Input: part model. Units: mm. Frame: model coordinates. Coordinates: 2 decimals unless noted, no trailing zeros. Loops run counter-clockwise (first coordinate to the right, second up) from the corner with the lowest first, then second, coordinate; pieces in that order, holes last. Notation, with made-up numbers: (47.25, 57.25) -> (105.25, 57.25) arc R17 ccw to (105.25, 61.25) -> close; hole circle Ø7 at (-40, -37.5). An arc over 180 degrees is marked (long way). Answer as a JSON object with one key per item and string values.
from build123d import *

# Parameters (mm, degrees)
SKETCH2_W               = 60.452
SKETCH2_H               = 3.175
BOSS_EXTRUDE3_DEPTH     = 2.54
CUT_EXTRUDE2_DEPTH      = 361.893602522
CUT_EXTRUDE2_DEPTH_BACK = 361.893602522
SKETCH4_W               = 60.325
SKETCH4_H               = 3.175
SKETCH4_W_2             = 3.175
SKETCH4_H_2             = 31.75


with BuildPart() as part:
    # Sketch2 → Boss-Extrude3 (new body)
    with BuildSketch(Plane.XY):
        Polygon((-213.36, -244.2845), (-213.36, -263.2075), (-213.36, -269.6845), (-113.03, -269.6845), (-113.03, -244.2845), (132.334, -244.2845), (132.334, -241.1095), (192.786, -241.1095), (192.786, -244.2845), (213.36, -244.2845), (239.808280092, -244.2845), (239.808280092, -147.0025), (213.36, -147.0025), (213.36, 147.0025), (239.808280092, 147.0025), (239.808280092, 244.2845), (213.36, 244.2845), (192.786, 244.2845), (192.786, 241.1095), (132.334, 241.1095), (132.334, 244.2845), (-113.03, 244.2845), (-113.03, 269.6845), (-213.36, 269.6845), (-213.36, 244.2845), align=None)
        with Locations((-162.56, -242.697)):
            Rectangle(SKETCH2_W, SKETCH2_H, mode=Mode.SUBTRACT)
        with Locations((-162.56, 242.697)):
            Rectangle(SKETCH2_W, SKETCH2_H, mode=Mode.SUBTRACT)
    extrude(amount=BOSS_EXTRUDE3_DEPTH)

    # Sketch4 → Cut-Extrude2 (cut, two sides: drawn at the far end of the back side and taken through both)
    with BuildSketch(Plane.XY.offset(2.54).offset(-CUT_EXTRUDE2_DEPTH_BACK)):
        with Locations((-162.6235, -145.542)):
            Rectangle(SKETCH4_W, SKETCH4_H)
        with Locations((-162.6235, -48.471666667)):
            Rectangle(SKETCH4_W, SKETCH4_H)
        with Locations((-162.6235, 48.598666667)):
            Rectangle(SKETCH4_W, SKETCH4_H)
        with Locations((-162.6235, 145.669)):
            Rectangle(SKETCH4_W, SKETCH4_H)
        with Locations((162.6235, -145.542)):
            Rectangle(SKETCH4_W, SKETCH4_H)
        with Locations((162.6235, -48.471666667)):
            Rectangle(SKETCH4_W, SKETCH4_H)
        with Locations((162.6235, 48.598666667)):
            Rectangle(SKETCH4_W, SKETCH4_H)
        with Locations((162.6235, 145.669)):
            Rectangle(SKETCH4_W, SKETCH4_H)
        with Locations((211.7725, -194.056)):
            Rectangle(SKETCH4_W_2, SKETCH4_H_2)
        with Locations((211.7725, -97.028)):
            Rectangle(SKETCH4_W_2, SKETCH4_H_2)
        with Locations((211.7725, 0)):
            Rectangle(SKETCH4_W_2, SKETCH4_H_2)
        with Locations((211.7725, 97.028)):
            Rectangle(SKETCH4_W_2, SKETCH4_H_2)
        with Locations((211.7725, 194.056)):
            Rectangle(SKETCH4_W_2, SKETCH4_H_2)
        with Locations((-211.7725, -97.028)):
            Rectangle(SKETCH4_W_2, SKETCH4_H_2)
        with Locations((-211.7725, 0)):
            Rectangle(SKETCH4_W_2, SKETCH4_H_2)
        with Locations((-211.7725, -194.056)):
            Rectangle(SKETCH4_W_2, SKETCH4_H_2)
        with Locations((-211.7725, 97.028)):
            Rectangle(SKETCH4_W_2, SKETCH4_H_2)
        with Locations((-211.7725, 194.056)):
            Rectangle(SKETCH4_W_2, SKETCH4_H_2)
    extrude(amount=CUT_EXTRUDE2_DEPTH + CUT_EXTRUDE2_DEPTH_BACK, mode=Mode.SUBTRACT)


solid = part.part
1. Line query: line 1 along Y through (x, z) = (180.5, 0.8); line 2 along X through (y, z) = (48, 2); line 3 along Y through (x, z) = (103.5, 0.65). Output: solid intervals per line, ascending.
Reply:
{"line 1": "y = -241.11 to -147.13, -143.95 to -50.06, -46.88 to 47.01, 50.19 to 144.08, 147.26 to 241.11", "line 2": "x = -213.36 to -192.79, -132.46 to 132.46, 192.79 to 213.36", "line 3": "y = -244.28 to 244.28"}
2. Section query B-B (x = 185.5). Return loops of the section in (y, z), plus the area to 3 significant figures.
Reply:
{"outline": "(-241.11, 0) -> (-147.13, 0) -> (-147.13, 2.54) -> (-241.11, 2.54) -> close; (-143.95, 0) -> (-50.06, 0) -> (-50.06, 2.54) -> (-143.95, 2.54) -> close; (-46.88, 0) -> (47.01, 0) -> (47.01, 2.54) -> (-46.88, 2.54) -> close; (50.19, 0) -> (144.08, 0) -> (144.08, 2.54) -> (50.19, 2.54) -> close; (147.26, 0) -> (241.11, 0) -> (241.11, 2.54) -> (147.26, 2.54) -> close", "area": "1,190 mm2"}
3. Section query C-C (z = 0.7). Count the separate pieces of the cut face and the enclosed holes in it, plus the area to 3 significant figures.
Reply:
{"separate pieces": "1", "enclosed holes": "12", "area": "215,000 mm2"}
4. Section query D-D (y = -74). Return loops of the section in (x, z), plus the area to 3 significant figures.
Reply:
{"outline": "(-213.36, 0) -> (213.36, 0) -> (213.36, 2.54) -> (-213.36, 2.54) -> close", "area": "1,080 mm2"}
5. Pin query (flat end, axial travel): P1, Ø1.3, axis at x = 212.5, z = 1, coming from the +Y side; P2, Ø1.3, axis at x = 174, z = 2, coming from the -Y side; P3, Ø1.3, axis at x = 212, z = 2, coming from the -Y side. Return the tip coordinate at first contact, or that it passes through.
Reply:
{"P1": "stops at y = 244.28", "P2": "stops at y = -241.11", "P3": "stops at y = -244.28"}
6. Section query A-A (x = -164.5). Return loops of the section in (y, z).
Reply:
{"outline": "(-269.68, 0) -> (-244.28, 0) -> (-244.28, 2.54) -> (-269.68, 2.54) -> close; (-241.11, 0) -> (-147.13, 0) -> (-147.13, 2.54) -> (-241.11, 2.54) -> close; (-143.95, 0) -> (-50.06, 0) -> (-50.06, 2.54) -> (-143.95, 2.54) -> close; (-46.88, 0) -> (47.01, 0) -> (47.01, 2.54) -> (-46.88, 2.54) -> close; (50.19, 0) -> (144.08, 0) -> (144.08, 2.54) -> (50.19, 2.54) -> close; (147.26, 0) -> (241.11, 0) -> (241.11, 2.54) -> (147.26, 2.54) -> close; (244.28, 0) -> (269.68, 0) -> (269.68, 2.54) -> (244.28, 2.54) -> close"}
